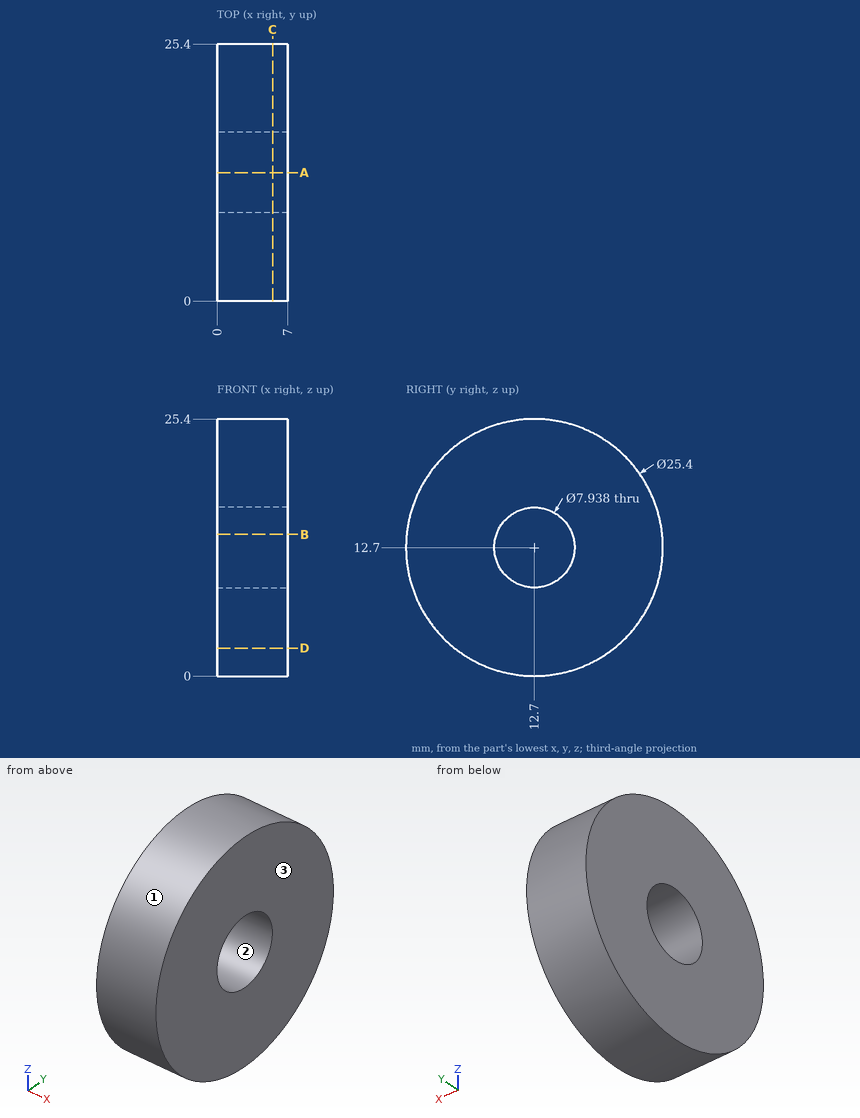
For this review, use the dimensioned drawing (mm, ordinates from the lowest corner) and the shaded views. Give positions to 0.01 mm unless a question says otherwise; leave off trailing zeros. Order: outer loops, then holes, each group sorted by start corner. A loop starts at its lowest first (then second) coordinate and runs counter-clockwise, first axis right, second up.
1) Take a section at B-B (z = 14). Give the boundary of the cut face in (x, y).
2) Wall thickness on line 1 (Y direction, x = 2.5, z = 12.7); line 2 (Z direction, x = 2.5, y = 12.5); line 3 (Z direction, x = 4.5, y = 14.75) (1 decimal): over which ranges is each line inside the solid? List them lowest first.
3) Take a section at C-C (x = 5.5). Give the boundary of the cut face in (y, z), then the cut area to 3 significant figures.
4) Insertion check: pin 1 (1.5 mm diameter, centred on x = 3, y = 8.5, fed in from -Z); pin 2 (1.5 mm diameter, centred on x = 1, z = 21.5, fed in from -Y); pin 3 (1 mm diameter, centred on x = 3.5, y = 12.5, fed in from -Z); pin 4 (1 mm diameter, centred on x = 4.5, y = 16, fed in from -Z). Each pin has a flat end and moves straight along its axis. Give the tip position at first contact, or say it passes through.
5) The part is to be moulded in two halves that separate along Y. For the marked faces 1, 2 and 3, say which applies: released by +Y, released by -Y, zero draft, split by the parting line, or undercut.
6) Take a section at D-D (z = 2.75). Give the boundary of the cut face in (x, y).
7) Take a section at A-A (y = 12.7). Give the boundary of the cut face in (x, z).
Derived:
1. outline: (0, 0.07) - (7, 0.07) - (7, 8.95) - (0, 8.95) - close; (0, 16.45) - (7, 16.45) - (7, 25.33) - (0, 25.33) - close
2. line 1: y = 0 to 8.73, 16.67 to 25.4
2. line 2: z = 0 to 8.74, 16.66 to 25.4
2. line 3: z = 0.2 to 9.3, 16.1 to 25.2
3. outline: circle Ø25.4 at (12.7, 12.7); hole circle Ø7.94 at (12.7, 12.7)
3. area: 457 mm2
4. pin 1: stops at z = 0.48
4. pin 2: stops at y = 2.88
4. pin 3: stops at z = 0
4. pin 4: stops at z = 0.31
5. face 1: split by the parting line
5. face 2: undercut
5. face 3: zero draft
6. outline: (0, 4.81) - (7, 4.81) - (7, 20.59) - (0, 20.59) - close
7. outline: (0, 0) - (7, 0) - (7, 8.73) - (0, 8.73) - close; (0, 16.67) - (7, 16.67) - (7, 25.4) - (0, 25.4) - close
